```python
from build123d import *

# Parameters (mm, degrees)
BASENUT_DEPTH   = 5.3
SKETCH3_R       = 1.7
HOLE_DEPTH      = 6.3
ENDCHAMFER_SIZE = 0.485714286


with BuildPart() as part:
    # Sketch1 → BaseNut (new body)
    with BuildSketch(Plane.XY):
        Polygon((2.309401077, -4), (4.618802154, 0), (2.309401077, 4), (-2.309401077, 4), (-4.618802154, 0), (-2.309401077, -4), align=None)
    extrude(amount=-BASENUT_DEPTH)

    # Sketch2 → Double-Chamfer (revolve, cut)
    with BuildSketch(Plane(origin=(0.481162538, 0, -5.099964691), x_dir=(0, 0, -1), z_dir=(0, -1, 0))):
        Polygon((-0.115823776, 4.137639616), (0.200035309, 4.137639616), (0.200035309, 2.958837462), align=None)
        Polygon((-5.099964691, 4.137639616), (-3.639964691, 4.137639616), (-5.099964691, 3.518837462), align=None)
    revolve(axis=Axis((0, 0, -4.462865094), (0, 0, 1)), mode=Mode.SUBTRACT)

    # Sketch3 → Hole (cut, through all)
    with BuildSketch(Plane.XY):
        Circle(SKETCH3_R)
    extrude(amount=-HOLE_DEPTH, mode=Mode.SUBTRACT)

    # EndChamfer
    endchamfer_edges = [part.edges().sort_by_distance(p)[0] for p in [
        (-1.7, 0, -5.3),
    ]]
    chamfer(endchamfer_edges, length=ENDCHAMFER_SIZE)


solid = part.part
```
The listing builds one solid part. Answer for the finished solid, in the listing's coordinates (mm). Coordinates: 2 decimals unless noted, no trailing zeros. Order: outer loops, then holes, each group sorted by start corner. A loop starts at its lowest first (then second) coordinate and runs counter-clockwise, first axis right, second up. Notation, with made-up numbers: M 23.5,-20 L 48.5,-20 A24 ccw 48.5,19 Z; hole C 38,-6.75 d7. An arc over 180 degrees is marked long. Answer as a JSON object with one key per item and string values. Group by question number.
1. Flat-ended cylindrical pins translate along their axes: P1, Ø1, axis at x = -3, y = 3, coming from the -Z side; P2, Ø1.5, axis at y = -3, z = -2, coming from the +X side. Find the tip coordinate at first contact, or state that the pin passes through.
2. Straight lines are drawn through the part: line 1 (Y direction, x = 0, z = -2.65); line 2 (X direction, y = -1, z = -0.7); line 3 (X direction, y = 0.75, z = -2.05). For each, find the intervals that lie inside material, in ascending order.
3. Section A-A on z = -4.35 is taken. Write down the section's boundary in (x, y).
4. Determine the mould class of faces 1 (the conical face through (4.15, -0.01, -0.35)), 2 (the conical face through (-2.06, 3.6, -0.35)), 3 (the cylindrical face through (-0.37, -1.66, -2.37)), 4 (the flat face through (0, 4, -3)) for opening direction X: released by +X, released by -X, zero draft, split by the parting line, or undercut.
5. Section B-B on z = -0.7 is taken. Write down the section's boundary in (x, y).
Values follow:
{
 "1": {"P1": "z = -5.22", "P2": "x = 3.32"},
 "2": {"line 1": "-4 to -1.7, 1.7 to 4", "line 2": "-4.04 to -1.37, 1.37 to 4.04", "line 3": "-4.19 to -1.53, 1.53 to 4.19"},
 "3": {"outline": "M -4.62,0 L -2.31,-4 L 2.31,-4 L 4.62,0 L 2.31,4 L -2.31,4 Z; hole C 0,0 d3.4"},
 "4": {"face 1": "released by +X", "face 2": "released by -X", "face 3": "undercut", "face 4": "zero draft"},
 "5": {"outline": "M -4.25,-0.64 L -2.68,-3.36 A4.3 ccw -1.57,-4 L 1.57,-4 A4.3 ccw 2.68,-3.36 L 4.25,-0.64 A4.3 ccw 4.25,0.64 L 2.68,3.36 A4.3 ccw 1.57,4 L -1.57,4 A4.3 ccw -2.68,3.36 L -4.25,0.64 A4.3 ccw Z; hole C 0,0 d3.4"}
}
